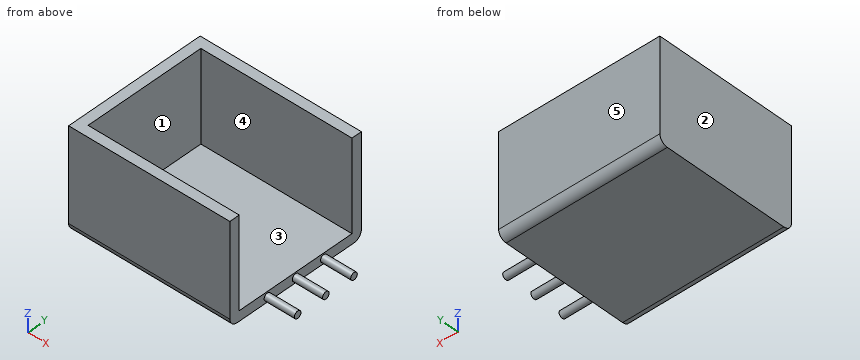
```python
from build123d import *

# Parameters (mm, degrees)
SKETCH1_W               = 150
SKETCH1_H               = 120
BOSS_EXTRUDE1_DEPTH     = 10
SKETCH2_R               = 3.5
BOSS_EXTRUDE2_DEPTH     = 30
CROQUIS2_W              = 100
CROQUIS2_H              = 120
SALIENTE_EXTRUIR1_DEPTH = 10
CROQUIS3_W              = 160
CROQUIS3_H              = 100
SALIENTE_EXTRUIR2_DEPTH = 10
CROQUIS4_W              = 160
CROQUIS4_H              = 100
SALIENTE_EXTRUIR3_DEPTH = 10
FILLET1_R               = 8


with BuildPart() as part:
    # Sketch1 → Boss-Extrude1 (new body)
    with BuildSketch(Plane.XY):
        with Locations((-75, 0)):
            Rectangle(SKETCH1_W, SKETCH1_H)
    extrude(amount=BOSS_EXTRUDE1_DEPTH)

    # Sketch2 → Boss-Extrude2 (add)
    with BuildSketch(Plane(origin=(0, 0, 0), x_dir=(0, 0, -1), z_dir=(1, 0, 0))):
        with Locations(Location((-5, 30, 0), (0, 0, 180))):
            Circle(SKETCH2_R)
        with Locations(Location((-5, -30, 0), (0, 0, 180))):
            Circle(SKETCH2_R)
        with Locations(Location((-5, 0, 0), (0, 0, 180))):
            Circle(SKETCH2_R)
    extrude(amount=BOSS_EXTRUDE2_DEPTH)

    # Croquis2 → Saliente-Extruir1 (add)
    with BuildSketch(Plane.ZY.offset(150)):
        with Locations((50, 0)):
            Rectangle(CROQUIS2_W, CROQUIS2_H)
    extrude(amount=SALIENTE_EXTRUIR1_DEPTH)

    # Croquis3 → Saliente-Extruir2 (add)
    with BuildSketch(Plane.XZ.offset(60)):
        with Locations((-80, 50)):
            Rectangle(CROQUIS3_W, CROQUIS3_H)
    extrude(amount=SALIENTE_EXTRUIR2_DEPTH)

    # Croquis4 → Saliente-Extruir3 (add)
    with BuildSketch(Plane(origin=(0, 60, 0), x_dir=(1, 0, 0), z_dir=(0, 1, 0))):
        with Locations((-80, -50)):
            Rectangle(CROQUIS4_W, CROQUIS4_H)
    extrude(amount=SALIENTE_EXTRUIR3_DEPTH)

    # Fillet1
    fillet1_edges = [part.edges().sort_by_distance(p)[0] for p in [
        (-80, -70, 0),
        (-80, 70, 0),
    ]]
    fillet(fillet1_edges, radius=FILLET1_R)


solid = part.part
```
Design review of the part built by this model. Coordinates are the model's own, in mm. Face numbers are marked on the shaded views. A direction names the side the tool comes from. Round coordinates to 2 decimals unless told otherwise and drop trailing zeros. Write each loop counter-clockwise with the first axis right and the second up, starting at its lowest first coordinate (ties: lowest second). Pieces come first, ordered by that corner, then holes.
Item 1: We need section D-D on y = -30. Write out the cut boundary in (x, z), and give its area (3 significant figures).
Item 2: Clearance check with a flat-ended pin moving along its axis: pin 1 Ø8 at (y, z) = (-38.5, 75) entering from +X. State where the tip first meets the part, or that it passes through.
Item 3: For the marked faces 4 and 5, list the 3-axis set-ups (+Z, -Z, +X, -X, +Y, -Y) from which the entire face can be reached by the end or side of a thin tool; tool diameter is ignored.
Item 4: We need section C-C on x = -39.5. Write out the cut boundary in (y, z).
Item 5: For probe 1 along Y at (x, z) = (-69.5, 92); probe 2 along X at (y, z) = (-19, 69); probe 3 along Z at (x, y) = (-93, 30.5), list the stretches that pass through material, from the lowest coordinate up.
Item 6: We need section B-B on y = 52.5. Write out the cut boundary in (x, z).
Item 7: The part is to be moulded in two halves that separate along X. For the marked faces 1, 2 and 3, say which applies: +X half, -X half, draft (parallel to the pull), parting line (faces both ways), or undercut.
Item 8: We need section A-A on z = 49. Write out the cut boundary in (x, y), and give its area (3 significant figures).
Returned:
1. outline: (-160, 0) - (0, 0) - (0, 1.5) - (30, 1.5) - (30, 8.5) - (0, 8.5) - (0, 10) - (-150, 10) - (-150, 100) - (-160, 100) - close
1. area: 2,710 mm2
2. pin 1: stops at x = -150
3. face 4: +Z, +X
3. face 5: +Z, -Z, +X, -X, +Y
4. outline: (-70, 8) arc R8 ccw to (-62, 0) - (62, 0) arc R8 ccw to (70, 8) - (70, 100) - (60, 100) - (60, 10) - (-60, 10) - (-60, 100) - (-70, 100) - close
5. probe 1: y = -70 to -60, 60 to 70
5. probe 2: x = -160 to -150
5. probe 3: z = 0 to 10
6. outline: (-160, 0) - (0, 0) - (0, 10) - (-150, 10) - (-150, 100) - (-160, 100) - close
7. face 1: +X half
7. face 2: -X half
7. face 3: draft
8. outline: (-160, -70) - (0, -70) - (0, -60) - (-150, -60) - (-150, 60) - (0, 60) - (0, 70) - (-160, 70) - close
8. area: 4,400 mm2
